For this review, use the dimensioned drawing (mm, ordinates from the lowest corner) and the shaded views. A direction names the side the tool comes from. Coordinates: 2 decimals unless noted, no trailing zeros. Order: outer loops, then holes, each group sorted by start corner. A loop starts at its lowest first (then second) coordinate and runs counter-clockwise, first axis right, second up. Notation, with made-up numbers: M 22,-31 L 50,-31 A25 cw 50,-16 Z; hole C 83.25,51.25 d6. An arc over 180 degrees is marked long. One line per item, written item: value.
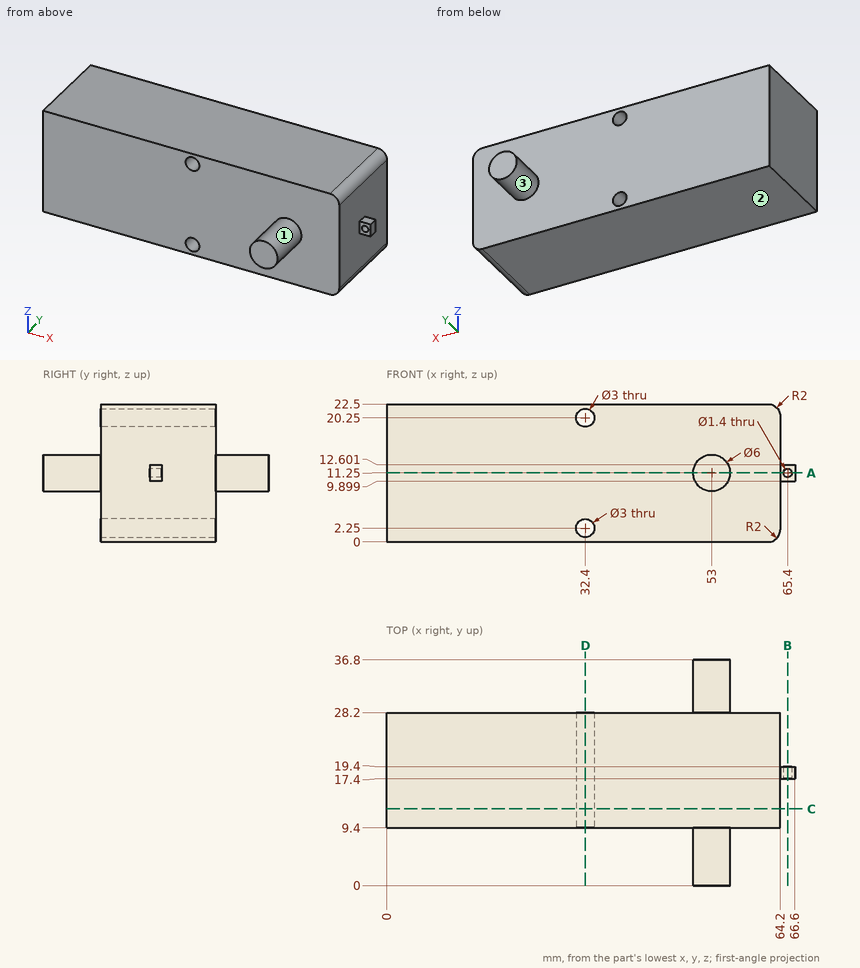
(1) Tool access review of the marked faces 1, 2 and 3: name each direction out of +Z, -Z, +X, -X, +Y, -Y from which nothing blocks a thin tool from reaching the whole face with its end or side.
Geometry results:
face 1: -Y
face 2: -Z, +X, -X, +Y, -Y
face 3: +Y
(2) We need section D-D, the plane x = 32.4. State the section outline as (y, z) points.
Geometry results:
outline: M 9.4,0 L 28.2,0 L 28.2,0.75 L 9.4,0.75 Z; M 9.4,3.75 L 28.2,3.75 L 28.2,18.75 L 9.4,18.75 Z; M 9.4,21.75 L 28.2,21.75 L 28.2,22.5 L 9.4,22.5 Z
(3) We need section B-B, the plane x = 65.4. State the section outline as (y, z) points.
Geometry results:
outline: M 17.4,9.9 L 19.4,9.9 L 19.4,10.55 L 17.4,10.55 Z; M 17.4,11.95 L 19.4,11.95 L 19.4,12.6 L 17.4,12.6 Z
(4) We need section C-C, the plane y = 12.5. State the section outline as (x, z) points.
Geometry results:
outline: M 0,0 L 62.2,0 A2 ccw 64.2,2 L 64.2,20.5 A2 ccw 62.2,22.5 L 0,22.5 Z; hole C 32.4,2.25 d3; hole C 32.4,20.25 d3
(5) Insertion check: pin 1 Ø7 at (x, z) = (29, 6.5) entering from +Y; pin 2 Ø6 at (y, z) = (23, 15.5) entering from +X; pin 3 Ø1.8 at (x, z) = (32.4, 20.25) entering from -Y; pin 4 Ø5 at (x, z) = (32.4, 2.25) entering from -Y. Each pin has a flat end and moves straight along its axis. Give the tip position at first contact, or say it passes through.
Geometry results:
pin 1: stops at y = 28.2
pin 2: stops at x = 64.2
pin 3: passes through
pin 4: stops at y = 9.4
(6) For L1, parallel to X at y = 18.3, z = 11.25; L2, parallel to X at y = 26.5, z = 2.25; L3, parallel to Z at x = 32, y = 15 (1 decimal), list the stretches that pass through material, from the lowest coordinate up.
Geometry results:
L1: x = 0 to 64.7, 66.1 to 66.6
L2: x = 0 to 30.9, 33.9 to 64.2
L3: z = 0 to 0.8, 3.7 to 18.8, 21.7 to 22.5
(7) We need section A-A, the plane z = 11.25. State the section outline as (x, y) points, plus the area to 3 significant figures.
Geometry results:
outline: M 0,9.4 L 50,9.4 L 50,0 L 56,0 L 56,9.4 L 64.2,9.4 L 64.2,17.4 L 64.7,17.4 L 64.7,19.4 L 64.2,19.4 L 64.2,28.2 L 56,28.2 L 56,36.8 L 50,36.8 L 50,28.2 L 0,28.2 Z; M 66.1,17.4 L 66.6,17.4 L 66.6,19.4 L 66.1,19.4 Z
area: 1,320 mm2
